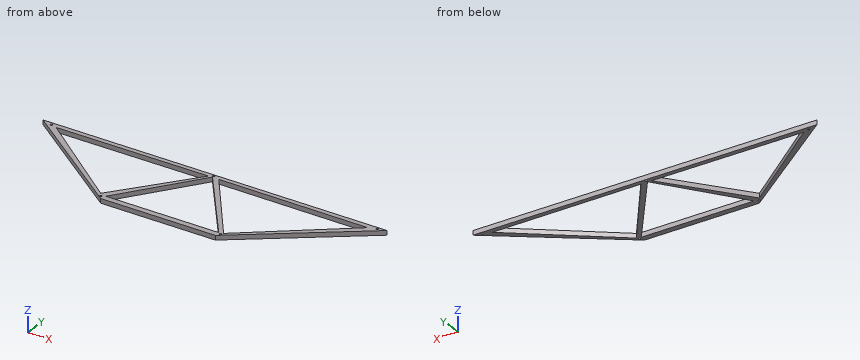
```python
from build123d import *

# Parameters (mm, degrees)
BOSS_EXTRUDE2_DEPTH = 15.61
CUT_EXTRUDE1_DEPTH  = 672.00199113
CUT_EXTRUDE2_DEPTH  = 672.00199113
SKETCH7_R           = 3.9
CUT_EXTRUDE3_DEPTH  = 672.00199113


with BuildPart() as part:
    # Sketch2 → Boss-Extrude2 (new body)
    with BuildSketch(Plane.XY):
        Polygon((-200, 0), (200, 0), (600, 300), (-600, 300), align=None)
    extrude(amount=BOSS_EXTRUDE2_DEPTH)

    # Sketch3 → Cut-Extrude1 (cut, through all)
    with BuildSketch(Plane.XY.offset(15.61)):
        Polygon((-195, 19.678308093), (198.68730415, 19.678308093), (0, 286.78421274), align=None)
    extrude(amount=-CUT_EXTRUDE1_DEPTH, mode=Mode.SUBTRACT)

    # Sketch5 → Cut-Extrude2 (cut, through all)
    with BuildSketch(Plane.XY.offset(15.61)):
        Polygon((-217.434189149, 26.151043002), (-12.810282728, 285.331439802), (-543.331948452, 283.448560198), align=None)
        Polygon((543.539861229, 283.448560198), (22.85265332, 285.331439802), (213.236522938, 23.158727928), align=None)
    extrude(amount=-CUT_EXTRUDE2_DEPTH, mode=Mode.SUBTRACT)

    # Sketch7 → Cut-Extrude3 (cut, through all)
    with BuildSketch(Plane.XY.offset(15.61)):
        with Locations((-563.626982451, 289.376274745)):
            Circle(SKETCH7_R)
        with Locations((0, 293.39210637)):
            Circle(SKETCH7_R)
        with Locations((571.769930615, 291.724280099)):
            Circle(SKETCH7_R)
        with Locations((208.154539122, 14.26724781)):
            Circle(SKETCH7_R)
        with Locations((-208.717094574, 13.075521501)):
            Circle(SKETCH7_R)
    extrude(amount=-CUT_EXTRUDE3_DEPTH, mode=Mode.SUBTRACT)


solid = part.part
```
Geometry: final body of the model. Coordinates: model frame, mm. Round coordinates to 2 decimals unless told otherwise and drop trailing zeros. Order: outer loops, then holes, each group sorted by start corner. A loop starts at its lowest first (then second) coordinate and runs counter-clockwise, first axis right, second up. Notation, with made-up numbers: (-34, 0.25) - (-21, 0.25) arc R20 ccw to (-21, 13.25) - close; hole circle Ø1 at (27.5, 32). An arc over 180 degrees is marked (long way). Use CSV: the item, a comma, the result in double quotes. Start each with the question number.
Q1. Section query A-A (x = 275.5). Return loops of the section in (y, z) (3 decimals).
Q2. Material intervals for line 1 along X through (y, z) = (85, 2.25); line 2 along X through (y, z) = (249, 6); line 3 along Y through (x, z) = (0, 10.5), sorted ascending. Write a range as from..to.
Q3. Section query B-B (y = 88). Return loops of the section in (x, z), and give its area (3 significant figures).
Q4. Section query D-D (x = -155.5). Return loops of the section in (y, z).
Q5. Section query C-C (z = 11.5). State how many separate pieces and enclosed holes the cut face has, and give its area (3 significant figures).
Q6. First-contact query: pin 1 (8 mm diameter, centred on y = 36.5, z = 5.5, fed in from +X); pin 2 (6 mm diameter, centred on x = 131, z = 11.5, fed in from -Y); pin 3 (4 mm diameter, centred on y = 71.5, z = 12.5, fed in from +X); pin 4 (1.5 mm diameter, centred on y = 47.5, z = 7, fed in from -X). Flat tips, straight axial feed; report the tip coordinate or a pass-through.
Result set:
1,outline,"(56.625, 0) - (72.224, 0) - (72.224, 15.61) - (56.625, 15.61) - close; (284.418, 0) - (300, 0) - (300, 15.61) - (284.418, 15.61) - close"
2,line 1,"x = -313.33..-291.97, -170.97..-147.31, 150.1..168.33, 291.71..313.33"
2,line 2,"x = -532..-499.7, -41.49..-27.58, 28.11..49.24, 499.83..532"
2,line 3,"y = 0..19.68, 286.78..289.49, 297.29..300"
3,outline,"(-317.33, 0) - (-295.77, 0) - (-295.77, 15.61) - (-317.33, 15.61) - close; (-168.6, 0) - (-145.12, 0) - (-145.12, 15.61) - (-168.6, 15.61) - close; (147.87, 0) - (166.15, 0) - (166.15, 15.61) - (147.87, 15.61) - close; (295.52, 0) - (317.33, 0) - (317.33, 15.61) - (295.52, 15.61) - close"
3,area,"1,330 mm2"
4,outline,"(0, 0) - (19.68, 0) - (19.68, 15.61) - (0, 15.61) - close; (73.78, 0) - (104.6, 0) - (104.6, 15.61) - (73.78, 15.61) - close; (284.83, 0) - (300, 0) - (300, 15.61) - (284.83, 15.61) - close"
5,separate pieces,"1"
5,enclosed holes,"8"
5,area,"50,500 mm2"
6,pin 1,"stops at x = 254"
6,pin 2,"stops at y = 0"
6,pin 3,"stops at x = 298"
6,pin 4,"stops at x = -264.33"
